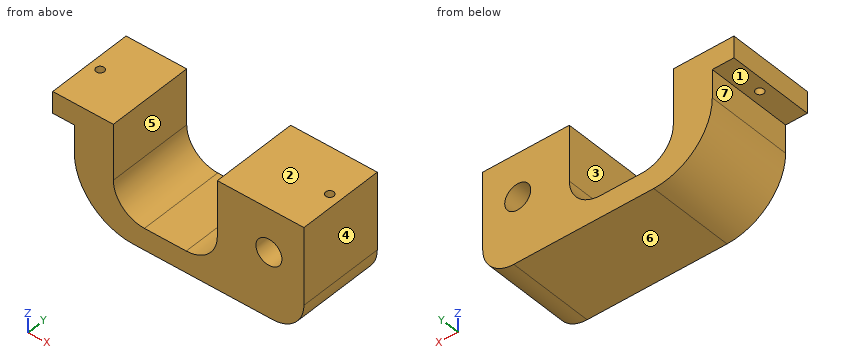
Autodesk Inventor part; units mm, degrees
ref_plane "YZ Plane" through (0, 0, 0) normal (1, 0, 0) x (0, 1, 0)
ref_plane "XZ Plane" through (0, 0, 0) normal (0, 1, 0) x (-1, 0, 0)
ref_plane "XY Plane" through (0, 0, 0) normal (0, 0, 1) x (1, 0, 0)
sketch "Sketch1" plane through (0, 0, 0) normal (0, 1, 0) x (-1, 0, 0)
  line L0 (4.35, -5) -> (-7.65, -5)
  line L1 (-7.65, -5) -> (-7.65, 5)
  line L2 (-7.65, 5) -> (4.35, 5)
  line L3 (4.35, 5) -> (4.35, -5)
  line L4 (4.35, -5) -> (-7.65, 5) construction
  line L5 (-7.65, -5) -> (4.35, 5) construction
  line L6 (4.35, 5) -> (11.35, 5)
  line L7 (11.35, 5) -> (11.35, 2.5)
  line L8 (11.35, 2.5) -> (8.85, 2.5)
  line L9 (8.85, 2.5) -> (8.85, -7.5)
  line L10 (-7.45, -7.5) -> (8.85, -7.5)
  line L11 (-7.65, 5) -> (-7.45, 5)
  line L12 (-17.65, 5) -> (-17.65, -7.5)
  line L13 (-17.65, -7.5) -> (-7.45, -7.5)
  line L14 (-17.65, 5) -> (-7.45, 5)
  circle A0 centre (-13.61, 0) radius 1.5
  dimension "d29" = 10
  dimension "d30" = 7
  dimension "d31" = 2.5
  dimension "d32" = 2.5
  dimension "d33" = 10
  dimension "d34" = 90
  dimension "d40" = 12
  dimension "d70" = 3
extrude "Extrusion9" add sketch "Sketch1" against normal blind 10 contours L3 L6 L7 L8 L9 L10 L13 L12 L14 L1 L0
fillet "Fillet7" radius 3.5875 2 edges at (-4.35, -5, -5) (7.65, -5, -5)
fillet "Fillet9" radius 3.5875 1 edges at (17.65, -5, -7.5)
fillet "Fillet10" radius 6.7625 1 edges at (-8.85, -5, -7.5)
sketch "Sketch5" plane through (-11.35, -10, 2.5) normal (0, 0, -1) x (-1, 0, 0)
  line L0 (-0.5, 0) -> (-0.5, 10)
  point P0 (-11.35, 10)
  point P1 (-0.5, 5)
sketch "Sketch6" plane through (-8.85, 0, 2.5) normal (0, 0, -1) x (-1, 0, 0)
  line L0 (2.5, -10) -> (0, -10)
  point P0 (-8.85, 0)
  point P1 (1.25, -5)
hole "Hole1" at (-10.1, -5, 2.5) direction (0, 0, 1) diameter 0.9398 depth 3.65 tip angle 118
sketch "Sketch7" plane through (7.65, 0, 5) normal (0, 0, 1) x (1, 0, 0)
  point P0 (-7.65, 0)
  point P1 (8.75, -5)
hole "Hole2" at (16.4, -5, 5) direction (0, 0, -1) diameter 0.9398 depth 3.65 tip angle 118
properties part number "chassis3"
For this review, take the finished solid that the model builds, in its own axes (mm). Face numbers are marked on the shaded views. A direction names the side the tool comes from. Coordinates: 2 decimals unless noted, no trailing zeros. Loops run counter-clockwise (first coordinate to the right, second up) from the corner with the lowest first, then second, coordinate; pieces in that order, holes last. Notation, with made-up numbers: (-4.5, 21.5) - (7.5, 21.5) arc R29 ccw to (7.5, 59.5) - close; hole circle Ø11 at (3.25, 19.25). An arc over 180 degrees is marked (long way). Return JSON: item names as keys, results as strings.
Item 1: Insertion check: pin 1 (2 mm diameter, centred on x = -10, y = -6, fed in from -Z); pin 2 (6 mm diameter, centred on y = -8.5, z = -4.5, fed in from -X); pin 3 (1 mm diameter, centred on x = 5, z = -3, fed in from -Y); pin 4 (1.4 mm diameter, centred on x = 1, y = -5, fed in from +Z). Each pin has a flat end and moves straight along its axis. Give the tip position at first contact, or say it passes through.
Determined:
{"pin 1": "stops at z = 2.5", "pin 2": "stops at x = -8.81", "pin 3": "passes through", "pin 4": "stops at z = -5"}
Item 2: Take a section at C-C (z = 0). Give the boundary of the cut face in (x, y), then the cut area to 3 significant figures.
Determined:
{"outline": "(-8.85, -10) - (-4.35, -10) - (-4.35, 0) - (-8.85, 0) - close; (7.65, -10) - (12.11, -10) - (12.11, 0) - (7.65, 0) - close; (15.11, -10) - (17.65, -10) - (17.65, 0) - (15.11, 0) - close", "area": "115 mm2"}
Item 3: For line 1 (X direction, y = -5, z = 3.35); line 2 (X direction, y = -7.5, z = 3.75); line 3 (Y direction, x = 16.4, z = 2.15), list the stretches that pass through material, from the lowest coordinate up.
Determined:
{"line 1": "x = -11.35 to -10.57, -9.63 to -4.35, 7.65 to 15.93, 16.87 to 17.65", "line 2": "x = -11.35 to -4.35, 7.65 to 17.65", "line 3": "y = -10 to -5.47, -4.53 to 0"}
Item 4: Take a section at A-A (z = 4.25). Give the boundary of the cut face in (x, y), then the cut area to 3 significant figures.
Determined:
{"outline": "(-11.35, -10) - (-4.35, -10) - (-4.35, 0) - (-11.35, 0) - close; (7.65, -10) - (17.65, -10) - (17.65, 0) - (7.65, 0) - close; hole circle Ø0.94 at (-10.1, -5); hole circle Ø0.94 at (16.4, -5)", "area": "169 mm2"}
Item 5: Take a section at B-B (x = -10.1). Give the boundary of the cut face in (y, z), then the cut area to 3 significant figures.
Determined:
{"outline": "(-10, 2.5) - (-5.47, 2.5) - (-5.47, 5) - (-10, 5) - close; (-4.53, 2.5) - (0, 2.5) - (0, 5) - (-4.53, 5) - close", "area": "22.7 mm2"}
Item 6: Mouldability with a two-part tool opening along X and no side actions: class the marked faces 4, 5, 6 and 7 as pulls with the +X half, pulls with the -X half, needs draft (parallel to the pull), parting line crosses it, or undercut.
Determined:
{"face 4": "pulls with the +X half", "face 5": "undercut", "face 6": "needs draft", "face 7": "pulls with the -X half"}
Item 7: For the marked faces 1, 2 and 3, list the 3-axis set-ups (+Z, -Z, +X, -X, +Y, -Y) from which the entire face can be reached by the end or side of a thin tool; tool diameter is ignored.
Determined:
{"face 1": "-Z, -X, +Y, -Y", "face 2": "+Z, +X, -X, +Y, -Y", "face 3": "+Z, +Y, -Y"}
